from build123d import *

# Parameters (mm, degrees)
SKETCH1_W                       = 50
SKETCH1_H                       = 95
BOSS_EXTRUDE1_DEPTH             = 9.525
TAP_DRILL_FOR_M4X0_7_TAP1_D     = 3.3
TAP_DRILL_FOR_M4X0_7_TAP1_DEPTH = 3.2
TAP_DRILL_FOR_M4X0_7_TAP1_TIP   = 0.991420021
TAP_DRILL_FOR_M4X0_7_TAP2_D     = 3.3
TAP_DRILL_FOR_M4X0_7_TAP2_DEPTH = 3.2
TAP_DRILL_FOR_M4X0_7_TAP2_TIP   = 0.991420021


with BuildPart() as part:
    # Sketch1 → Boss-Extrude1 (new body)
    with BuildSketch(Plane.XY):
        Rectangle(SKETCH1_W, SKETCH1_H)
    extrude(amount=-BOSS_EXTRUDE1_DEPTH)

    # Tap Drill for M4x0.7 Tap1
    with Locations(Plane.XZ.offset(47.5)):
        with Locations((16.67, -4.7625), (0, -4.7625), (-16.67, -4.7625)):
            Hole(TAP_DRILL_FOR_M4X0_7_TAP1_D / 2, depth=TAP_DRILL_FOR_M4X0_7_TAP1_DEPTH)
            with Locations((0, 0, -(TAP_DRILL_FOR_M4X0_7_TAP1_DEPTH + TAP_DRILL_FOR_M4X0_7_TAP1_TIP / 2))):  # 118° drill point
                Cone(0, TAP_DRILL_FOR_M4X0_7_TAP1_D / 2, TAP_DRILL_FOR_M4X0_7_TAP1_TIP, mode=Mode.SUBTRACT)

    # Tap Drill for M4x0.7 Tap2
    with Locations(Plane(origin=(0, 47.5, 0), x_dir=(1, 0, 0), z_dir=(0, 1, 0))):
        with Locations((0, 4.7625), (16.67, 4.7625), (-16.67, 4.7625)):
            Hole(TAP_DRILL_FOR_M4X0_7_TAP2_D / 2, depth=TAP_DRILL_FOR_M4X0_7_TAP2_DEPTH)
            with Locations((0, 0, -(TAP_DRILL_FOR_M4X0_7_TAP2_DEPTH + TAP_DRILL_FOR_M4X0_7_TAP2_TIP / 2))):  # 118° drill point
                Cone(0, TAP_DRILL_FOR_M4X0_7_TAP2_D / 2, TAP_DRILL_FOR_M4X0_7_TAP2_TIP, mode=Mode.SUBTRACT)


solid = part.part
Build history of the part. All positions in model axes, mm. A direction names the side the tool comes from. Round coordinates to 2 decimals unless told otherwise and drop trailing zeros. One line per question, with ' | ' between items.
1. Tool access for faces 5 (the face through (0.358, -45.878, -6.373)), 6 (the face through (0, -47.5, -7)), 7 (the face through (17.886, 45.878, -5.878)): list every direction of +Z, -Z, +X, -X, +Y, -Y with a clear straight run to the whole face (end or side of a thin tool).
Results are:
face 5: -Y | face 6: +Z, -Z, +X, -X, -Y | face 7: +Y
2. Mould opens along X. For faces 1 (the face through (16.384, -43.481, -4.75)), 2 (the face through (-25, -1, -5)), 3 (the face through (0, 1, 0)), 4 (the face through (-0.227, -43.481, -4.937)) say: released by +X, released by -X, zero draft, split by the parting line, or undercut.
Results are:
face 1: undercut | face 2: released by -X | face 3: zero draft | face 4: undercut
3. Drop flat-ended pins along their axis: pin 1 Ø3 at (x, z) = (16.67, -4.76) entering from -Y; pin 2 Ø5.5 at (x, z) = (16.67, -4.76) entering from -Y; pin 3 Ø2 at (x, z) = (0, -4.76) entering from +Y. Give the stop position or say it passes through.
Results are:
pin 1: y = -44.21 | pin 2: y = -47.5 | pin 3: y = 43.91
4. Drill centre lines: line 1 along Z through (x, y) = (-16.67, -46.1) (1 decimal); line 2 along Z through (x, y) = (16, -46) (3 decimals); line 3 along Y through (x, z) = (-16, -5.5). Where is each one in solid material? Low to high. Write a range as from..to.
Results are:
line 1: -9.5..-6.4, -3.1..0 | line 2: -9.525..-6.27, -3.255..0 | line 3: -43.91..43.91
